Work out the finished part from the listing and answer in its coordinate system (mm). Face numbers are marked on the shaded views. A direction names the side the tool comes from. Coordinates: 2 decimals unless noted, no trailing zeros. Write each loop counter-clockwise with the first axis right and the second up, starting at its lowest first coordinate (ties: lowest second). Pieces come first, ordered by that corner, then holes. Notation, with made-up numbers: M 87.25,62.25 L 118.25,62.25 A12 ccw 118.25,69.25 Z; hole C 22.25,60.5 d8. An arc over 180 degrees is marked long. Use CSV: the item, a comma, the result in double quotes.
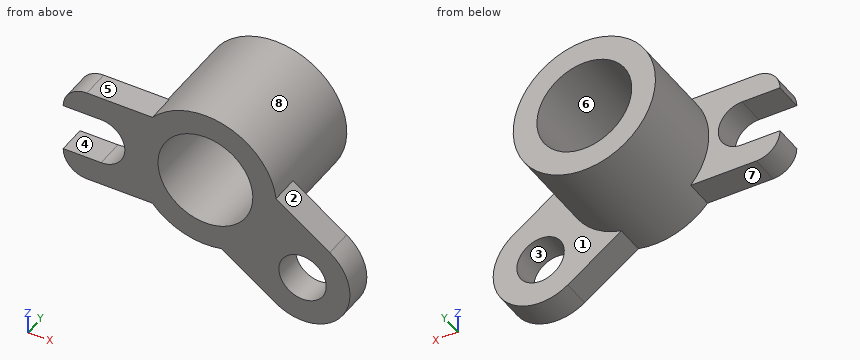
from build123d import *

# Parameters (mm, degrees)
SKETCH_1_R      = 15
SKETCH_1_R_2    = 10
EXTRUDE_1_DEPTH = 25
SKETCH_2_R      = 5
EXTRUDE_2_DEPTH = 6


with BuildPart() as part:
    # 草圖1 → 伸長1 (new body)
    with BuildSketch(Plane(origin=(0, 0, 0), x_dir=(1, 0, 0), z_dir=(0, 1, 0))):
        with Locations(Location((0, 0, 0), (0, 0, 270))):
            Circle(SKETCH_1_R)
        with Locations(Location((0, 0, 0), (0, 0, 270))):
            Circle(SKETCH_1_R_2, mode=Mode.SUBTRACT)
    extrude(amount=EXTRUDE_1_DEPTH)

    # 草圖2 → 伸長2 (add)
    # profile 1 of 2: a face of its own
    with BuildSketch(Plane(origin=(0, 0, 0), x_dir=(1, 0, 0), z_dir=(0, 1, 0))):
        with BuildLine():
            ThreePointArc((-11.180339887, -10), (-15, 0), (-11.180339887, 10))
            Line((-11.180339887, 10), (-25, 10))
            ThreePointArc((-25, 10), (-28.535533906, 8.535533906), (-30, 5))
            Line((-30, 5), (-22, 5))
            ThreePointArc((-22, 5), (-17, 0), (-22, -5))
            Line((-22, -5), (-30, -5))
            ThreePointArc((-30, -5), (-28.535533906, -8.535533906), (-25, -10))
            Line((-25, -10), (-11.180339887, -10))
        make_face()
    # profile 2 of 2: a face of its own
    with BuildSketch(Plane(origin=(0, 0, 0), x_dir=(1, 0, 0), z_dir=(0, 1, 0))):
        with BuildLine():
            Line((14.743036744, 22.530931352), (3.422633911, 14.604299953))
            ThreePointArc((3.422633911, 14.604299953), (11.754563128, 9.318274822), (15, 0))
            ThreePointArc((15, 0), (14.973517282, -0.89094344), (14.894162638, -1.778740933))
            Line((14.894162638, -1.778740933), (26.214565471, 6.147890466))
            ThreePointArc((26.214565471, 6.147890466), (28.67032155, 20.075175272), (14.743036744, 22.530931352))
        make_face()
        with Locations(Location((20.478801107, 14.339410909, 0), (0, 0, 270))):
            Circle(SKETCH_2_R, mode=Mode.SUBTRACT)
    extrude(amount=EXTRUDE_2_DEPTH)


solid = part.part
Item 1: Consider probe 1 along X at (y, z) = (18.5, 0); probe 2 along Z at (x, y) = (-25, 2.75); probe 3 along Y at (x, z) = (7.5, -15.5). Determine where each line is inside the solid, lowest interval first.
Answer:
probe 1,"x = -15 to -10, 10 to 15"
probe 2,"z = -10 to -5, 5 to 10"
probe 3,"y = 0 to 6"
Item 2: Given pin 1 (9 mm diameter, centred on x = 20.48, z = -14.34, fed in from +Y); pin 2 (6 mm diameter, centred on y = 15.5, z = 5.5, fed in from -X); pin 3 (6 mm diameter, centred on y = 19, z = 0, fed in from -X); pin 4 (1.8 mm diameter, centred on x = -26.5, y = 2, fed in from +Z), each flat-ended and moving along its own axis, determine where each tip first touches the part or whether it passes through.
Answer:
pin 1,"passes through"
pin 2,"stops at x = -14.79"
pin 3,"stops at x = -15"
pin 4,"stops at z = 9.96"
Item 3: The part is cut by section C-C (y = 4.5). Write down the section's boundary in (x, z).
Answer:
outline,"M -30,-5 A5 ccw -25,-10 L -11.18,-10 A15 ccw 3.42,-14.6 L 14.74,-22.53 A10 ccw 26.21,-6.15 L 14.89,1.78 A15 ccw -11.18,10 L -25,10 A5 ccw -30,5 L -22,5 A5 cw -22,-5 Z; hole C 0,0 d20; hole C 20.48,-14.34 d10"
Item 4: The part is cut by section B-B (z = -18.5). Write down the section's boundary in (x, y), then the cut area to 3 significant figures.
Answer:
outline,"M 8.99,0 L 17.71,0 L 17.71,6 L 8.99,6 Z; M 23.25,0 L 29.57,0 L 29.57,6 L 23.25,6 Z"
area,"90.2 mm2"
Item 5: A tool of negligible diameter and unlimited length cuts with its end or side. For the marked faces 4, 5, 6, 7 and 8, from which of +Z, -Z, +X, -X, +Y, -Y can it reach the whole face along a straight path? Write none if from no direction.
Answer:
face 4,"-X, +Y, -Y"
face 5,"+Z, -X, +Y, -Y"
face 6,"+Y, -Y"
face 7,"-Z, -X, +Y, -Y"
face 8,"+Y"
Item 6: For a pull along X with two mould halves and no side action, classify the marked faces 1, 2 and 3 as released by +X, released by -X, zero draft, split by the parting line, or undercut.
Answer:
face 1,"zero draft"
face 2,"released by +X"
face 3,"undercut"
Item 7: The part is cut by section D-D (x = -12). Write down the section's boundary in (y, z), then the cut area to 3 significant figures.
Answer:
outline,"M 0,-10 L 6,-10 L 6,-9 L 25,-9 L 25,9 L 6,9 L 6,10 L 0,10 Z"
area,"462 mm2"
Item 8: The part is cut by section A-A (x = 0). Write down the section's boundary in (y, z), then the cut area to 3 significant figures.
Answer:
outline,"M 0,-15 L 25,-15 L 25,-10 L 0,-10 Z; M 0,10 L 25,10 L 25,15 L 0,15 Z"
area,"250 mm2"
